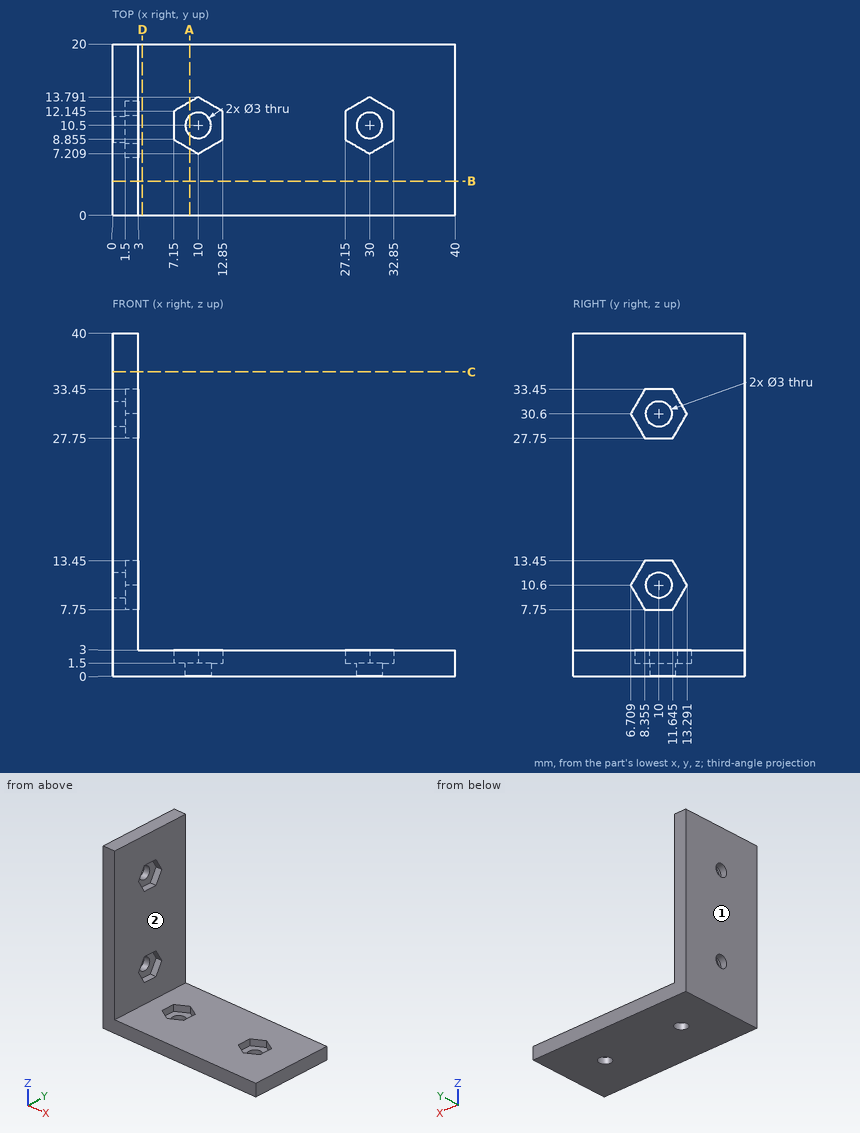
Could you check a few things on this drawing? It's one solid part, dimensions in mm from its lowest x, y, z. A direction names the side the tool comes from. Give positions to 0.01 mm unless a question says otherwise; leave off trailing zeros. Order: outer loops, then holes, each group sorted by start corner. A loop starts at its lowest first (then second) coordinate and runs counter-clockwise, first axis right, second up. Notation, with made-up numbers: (57.5, -20.5) - (64.5, -20.5) arc R23 ccw to (64.5, -5.5) - close; hole circle Ø10 at (7, -9). An arc over 180 degrees is marked (long way). One line per item, written item: value. Start each with the question number.
1. For the marked faces 1 and 2, which set-ups out of +Z, -Z, +X, -X, +Y, -Y let a thin tool reach every point of the face, with its end or its side?
2. Imagine slicing it at C-C on z = 35.5. List the corners of the cut face in (x, y) for me, plus the area to 3 significant figures.
3. Imagine slicing it at B-B on y = 4. List the corners of the cut face in (x, z) for me.
4. For P1, Ø12, axis at y = 10, z = 15.5, coming from the -X side; P2, Ø1.5, axis at x = 29.5, y = 10, coming from the +Z side; P3, Ø4.5, axis at x = 31, y = 9, coming from the +Z side; P4, Ø6.5, axis at y = 10.5, z = 30.5, coming from the +X side, each with a flat end and sliding along its axis, tell me the tip position at first contact or that it passes through.
5. If I drill on probe 1 along Y at (x, z) = (0.7, 10.6); probe 2 along X at (y, z) = (17.5, 33.5), over which ranges is the centre line in solid material (lowest first)?
6. Imagine slicing it at A-A on x = 9. List the corners of the cut face in (y, z) for me.
7. Imagine slicing it at D-D on x = 3.5. List the corners of the cut face in (y, z) for me.
Values:
1. face 1: +Z, -Z, -X, +Y, -Y
1. face 2: +Z, +X, +Y, -Y
2. outline: (0, 0) - (3, 0) - (3, 20) - (0, 20) - close
2. area: 60.0 mm²
3. outline: (0, 0) - (40, 0) - (40, 3) - (3, 3) - (3, 40) - (0, 40) - close
4. P1: x = 0
4. P2: through
4. P3: z = 3
4. P4: x = 3
5. probe 1: 0 to 8.5, 11.5 to 20
5. probe 2: 0 to 3
6. outline: (0, 0) - (9.38, 0) - (9.38, 1.5) - (7.79, 1.5) - (7.79, 3) - (0, 3) - close; (11.62, 0) - (20, 0) - (20, 3) - (13.21, 3) - (13.21, 1.5) - (11.62, 1.5) - close
7. outline: (0, 0) - (20, 0) - (20, 3) - (0, 3) - close
